from build123d import *

# Parameters (mm, degrees)
SKETCH1_W                              = 31.75
SKETCH1_H                              = 38.1
BOSS_EXTRUDE1_DEPTH                    = 20.6375
HOLE1_D                                = 22.225
TAPPED_HOLE_FOR_10_32_HELICOIL1_D      = 5.1054
TAPPED_HOLE_FOR_10_32_HELICOIL2_REACH  = 48.147
TAPPED_HOLE_FOR_10_32_HELICOIL2_BORE_R = 2.5527


with BuildPart() as part:
    # Sketch1 → Boss-Extrude1 (new, symmetric)
    with BuildSketch(Plane(origin=(0, 0, 0), x_dir=(0, 0, -1), z_dir=(1, 0, 0))):
        Rectangle(SKETCH1_W, SKETCH1_H)
    extrude(amount=BOSS_EXTRUDE1_DEPTH, both=True)

    # Hole1 (through all)
    with Locations(Plane.XY.offset(15.875)):
        with Locations((0, 3.175)):
            Hole(HOLE1_D / 2)

    # Tapped Hole for #10-32 Helicoil1 (through all)
    with Locations(Plane(origin=(0, 19.05, 0), x_dir=(1, 0, 0), z_dir=(0, 1, 0))):
        with Locations((-15.875, 0), (15.875, 0)):
            Hole(TAPPED_HOLE_FOR_10_32_HELICOIL1_D / 2)

    # Tapped Hole for #10-32 Helicoil2 bore → Tapped Hole for #10-32 Helicoil2 (cut, up to next)
    with BuildSketch(Plane(origin=(0, -19.05, 0), x_dir=(-1, 0, 0), z_dir=(0, -1, 0)), mode=Mode.PRIVATE) as tapped_hole_for_10_32_helicoil2_sk1:
        with Locations((0, 9.525)):
            Circle(TAPPED_HOLE_FOR_10_32_HELICOIL2_BORE_R)
    tapped_hole_for_10_32_helicoil2_tool1 = extrude(tapped_hole_for_10_32_helicoil2_sk1.sketch, amount=-TAPPED_HOLE_FOR_10_32_HELICOIL2_REACH, mode=Mode.PRIVATE) & part.part
    # Tapped Hole for #10-32 Helicoil2 bore → Tapped Hole for #10-32 Helicoil2 (cut, up to next)
    with BuildSketch(Plane(origin=(0, -19.05, 0), x_dir=(-1, 0, 0), z_dir=(0, -1, 0)), mode=Mode.PRIVATE) as tapped_hole_for_10_32_helicoil2_sk2:
        with Locations((0, -9.525)):
            Circle(TAPPED_HOLE_FOR_10_32_HELICOIL2_BORE_R)
    tapped_hole_for_10_32_helicoil2_tool2 = extrude(tapped_hole_for_10_32_helicoil2_sk2.sketch, amount=-TAPPED_HOLE_FOR_10_32_HELICOIL2_REACH, mode=Mode.PRIVATE) & part.part
    add(tapped_hole_for_10_32_helicoil2_tool1.solids().sort_by_distance((0, -19.05, -9.525))[0], mode=Mode.SUBTRACT)
    add(tapped_hole_for_10_32_helicoil2_tool2.solids().sort_by_distance((0, -19.05, 9.525))[0], mode=Mode.SUBTRACT)


solid = part.part
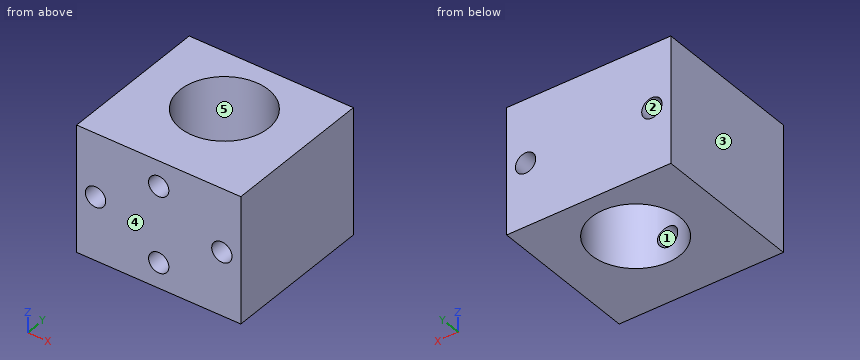
Geometry check sheet. Reference: the model listing, model coordinates, mm. Face numbers are marked on the shaded views. A direction names the side the tool comes from. Give positions to 0.01 mm unless a question says otherwise; leave off trailing zeros. Order: outer loops, then holes, each group sorted by start corner. A loop starts at its lowest first (then second) coordinate and runs counter-clockwise, first axis right, second up.
1. Sectioned sample at A-A (y = 4.5). Record the boundary of the cut face in (x, z) (1 decimal), then the cut area to 3 significant figures.
Completed:
outline: (-20.6, -15.9) - (-11, -15.9) - (-11, 15.9) - (-20.6, 15.9) - close; (11, -15.9) - (20.6, -15.9) - (20.6, 15.9) - (11, 15.9) - close; hole circle Ø5.1 at (-15.9, 0); hole circle Ø5.1 at (15.9, 0)
area: 569 mm2
2. Access from +Z, -Z, +X, -X, +Y, -Y to the whole of each face (thin tool, end or side, straight path). Record for the marked faces 1 and 2.
Completed:
face 1: -Y
face 2: +Y, -Y
3. Sectioned sample at B-B (z = 0). State how many separate pieces and enclosed holes the cut face has, then the cut area to 3 significant figures.
Completed:
separate pieces: 3
enclosed holes: 1
area: 796 mm2
4. Scan lines: line 1 (Z direction, x = 0, y = -14) (3 decimals); line 2 (Y direction, x = 0.5, z = 14); line 3 (X direction, y = 3, z = -0.5). Record each from-to range of solid material in increasing order.
Completed:
line 1: z = -15.875 to -12.078, -6.972 to 6.972, 12.078 to 15.875
line 2: y = -19.05 to -7.93, 14.28 to 19.05
line 3: x = -20.64 to -18.38, -13.37 to -11.11, 11.11 to 13.37, 18.38 to 20.64
5. Draft check along Y on the marked faces 3, 4 and 5. Enter one of: pulls with the +Y half, pulls with the -Y half, needs draft (parallel to the pull), parting line crosses it, or undercut.
Completed:
face 3: needs draft
face 4: pulls with the -Y half
face 5: undercut
6. Sectioned sample at D-D (y = 15). Record the boundary of the cut face in (x, z) (1 decimal), then the cut area to 3 significant figures.
Completed:
outline: (-20.6, -15.9) - (20.6, -15.9) - (20.6, 15.9) - (-20.6, 15.9) - close; hole circle Ø5.1 at (-15.9, 0); hole circle Ø5.1 at (15.9, 0)
area: 1,270 mm2
